Design review of the part built by this model. Coordinates are the model's own, in mm. A direction names the side the tool comes from. Coordinates: 2 decimals unless noted, no trailing zeros. Write each loop counter-clockwise with the first axis right and the second up, starting at its lowest first coordinate (ties: lowest second). Pieces come first, ordered by that corner, then holes. Notation, with made-up numbers: (-24, -26.75) - (15, -26.75) arc R20 ccw to (15, -7.75) - close; hole circle Ø1 at (25, -13.5). An arc over 180 degrees is marked (long way). Answer as CSV lines item,"result". Start each with the question number.
Q1. Clearance check with flat-ended pins moving along their axes: pin 1 (4 mm diameter, centred on x = 18.5, z = -5.5, fed in from -Y); pin 2 (2 mm diameter, centred on x = 8.5, y = 18, fed in from -Z); pin 3 (2 mm diameter, centred on x = -26, y = -31, fed in from +Z); pin 4 (3.5 mm diameter, centred on y = 29, z = -7.5, fed in from -X). State where each tip first meets the part, or that it passes through.
Q2. We need section A-A (x = 17.5). Write out the cut boundary in (y, z), plus the area to 3 significant figures.
Q3. We need section D-D (z = 3.5). Write out the cut boundary in (x, y), plus the area to 3 significant figures.
Q4. For line 1 along X through (y, z) = (17.5, 2.75); line 2 along Y through (x, z) = (15.5, -2.5); line 3 along X through (y, z) = (-26.5, -8), list the stretches that pass through material, from the lowest coordinate up. Write a range as [from, to].
Q5. Machinability: for faces 1 (the face through (25, -10, 3)), 2 (the face through (26, 22.85, -10)), 3 (the face through (9, -32, 0)), 4 (the face through (17, -31, -2)), 5 (the face through (-16.227, 31.299, -9.988)), which of the approach directions +Z, -Z, +X, -X, +Y, -Y give a long, thin tool a straight path to every point of the face, cutting with its end or side? Answer none if there is none.
Q6. We need section C-C (y = -15). Write out the cut boundary in (x, z), plus the area to 3 significant figures.
Q7. We need section B-B (z = -5.72). Write out the cut boundary in (x, y), plus the area to 3 significant figures.
Q8. Mouldability with a two-part tool opening along X and no side actions: class faces 6 (the face through (-26.373, 21.059, 3.131)), 7 (the face through (15, -30, 3)), 8 (the face through (-25, -11, 3)) as pulls with the +X half, pulls with the -X half, needs draft (parallel to the pull), parting line crosses it, or undercut.
from build123d import *

# Parameters (mm, degrees)
SKETCH1_R                                       = 2.85
BOSS_EXTRUDE1_DEPTH                             = 6.35
SKETCH2_W                                       = 25.4
SKETCH2_H                                       = 69.5
SKETCH2_W_2                                     = 14.7
SKETCH2_H_2                                     = 52.8
BOSS_EXTRUDE2_DEPTH                             = 15.578435
CSK_FOR_M8_FLAT_HEAD_MACHINE_SCREW1_D           = 9
CSK_FOR_M8_FLAT_HEAD_MACHINE_SCREW1_DEPTH       = 17.5
CSK_FOR_M8_FLAT_HEAD_MACHINE_SCREW1_CSINK_D     = 17.3
CSK_FOR_M8_FLAT_HEAD_MACHINE_SCREW1_CSINK_ANGLE = 90
CSK_FOR_M8_FLAT_HEAD_MACHINE_SCREW1_TIP         = 2.703872786
SKETCH6_W                                       = 15.578435
SKETCH6_H                                       = 11.9
BOSS_EXTRUDE3_DEPTH                             = 25.572145
SKETCH7_W                                       = 15.578435
SKETCH7_H                                       = 11.9
BOSS_EXTRUDE4_DEPTH                             = 10.937286
SKETCH8_R                                       = 2.5273
CUT_EXTRUDE1_DEPTH                              = 7
SKETCH9_W                                       = 10
SKETCH9_H                                       = 11.9
BOSS_EXTRUDE5_DEPTH                             = 4.972688
SKETCH10_R                                      = 2.5273
CUT_EXTRUDE2_DEPTH                              = 7
SKETCH11_W                                      = 5.3384196
SKETCH11_H                                      = 10
BOSS_EXTRUDE6_DEPTH                             = 5.35
SKETCH14_W                                      = 5.35
SKETCH14_H                                      = 10
CUT_EXTRUDE4_DEPTH                              = 5.33842
SKETCH15_W                                      = 5
SKETCH15_H                                      = 5
SKETCH15_W_2                                    = 8
SKETCH15_H_2                                    = 8
BOSS_EXTRUDE7_DEPTH                             = 8
SKETCH16_R                                      = 2.5273
CUT_EXTRUDE5_DEPTH                              = 7


with BuildPart() as part:
    # Sketch1 → Boss-Extrude1 (new body)
    with BuildSketch(Plane.XY):
        with BuildLine():
            Line((-5, 30), (5, 30))
            Line((5, 30), (25, 30))
            Line((25, 30), (25, 20.148215542))
            Line((25, 20.148215542), (27.91315613, 21.830127018))
            ThreePointArc((27.91315613, 21.830127018), (34.743283149, 19.999999999), (32.91315613, 13.16987298))
            Line((32.91315613, 13.16987298), (25, 8.601210158))
            Line((25, 8.601210158), (25, -30))
            Line((25, -30), (5.102267, -30))
            Line((5.102267, -30), (5.102267, -40))
            ThreePointArc((5.102267, -40), (0.102267, -45), (-4.897733, -40))
            Line((-4.897733, -40), (-4.897733, -30))
            Line((-4.897733, -30), (-25, -30))
            Line((-25, -30), (-25, 8.719297918))
            Line((-25, 8.719297918), (-32.70862213, 13.16987298))
            ThreePointArc((-32.70862213, 13.16987298), (-34.538749149, 19.999999999), (-27.70862213, 21.830127018))
            Line((-27.70862213, 21.830127018), (-25, 20.266303302))
            Line((-25, 20.266303302), (-25, 30))
            Line((-25, 30), (-5, 30))
        make_face()
        with Locations((0.102267, -40)):
            Circle(SKETCH1_R, mode=Mode.SUBTRACT)
        with Locations((30.41315613, 17.499999999)):
            Circle(SKETCH1_R, mode=Mode.SUBTRACT)
        with Locations((-30.20862213, 17.499999999)):
            Circle(SKETCH1_R, mode=Mode.SUBTRACT)
    extrude(amount=BOSS_EXTRUDE1_DEPTH)

    # Sketch2 → Boss-Extrude2 (add)
    with BuildSketch(Plane(origin=(0, 0, 0), x_dir=(-1, 0, 0), z_dir=(0, 0, -1))):
        Rectangle(SKETCH2_W, SKETCH2_H)
        with Locations((0, -3)):
            Rectangle(SKETCH2_W_2, SKETCH2_H_2, mode=Mode.SUBTRACT)
    extrude(amount=BOSS_EXTRUDE2_DEPTH)

    # CSK for M8 Flat Head Machine Screw1
    with Locations(Plane.XY.offset(6.35)):
        with Locations((0, -3)):
            CounterSinkHole(CSK_FOR_M8_FLAT_HEAD_MACHINE_SCREW1_D / 2, CSK_FOR_M8_FLAT_HEAD_MACHINE_SCREW1_CSINK_D / 2, depth=CSK_FOR_M8_FLAT_HEAD_MACHINE_SCREW1_DEPTH, counter_sink_angle=CSK_FOR_M8_FLAT_HEAD_MACHINE_SCREW1_CSINK_ANGLE)
            with Locations((0, 0, -(CSK_FOR_M8_FLAT_HEAD_MACHINE_SCREW1_DEPTH + CSK_FOR_M8_FLAT_HEAD_MACHINE_SCREW1_TIP / 2))):  # 118° drill point
                Cone(0, CSK_FOR_M8_FLAT_HEAD_MACHINE_SCREW1_D / 2, CSK_FOR_M8_FLAT_HEAD_MACHINE_SCREW1_TIP, mode=Mode.SUBTRACT)

    # Sketch6 → Boss-Extrude3 (add)
    with BuildSketch(Plane(origin=(12.7, 0, 0), x_dir=(0, 0, -1), z_dir=(1, 0, 0))):
        with Locations((7.7892175, 28.8)):
            Rectangle(SKETCH6_W, SKETCH6_H)
    extrude(amount=BOSS_EXTRUDE3_DEPTH)

    # Sketch7 → Boss-Extrude4 (add)
    with BuildSketch(Plane.ZY.offset(12.7)):
        with Locations((-7.7892175, 28.8)):
            Rectangle(SKETCH7_W, SKETCH7_H)
    extrude(amount=BOSS_EXTRUDE4_DEPTH)

    # Sketch8 → Cut-Extrude1 (cut)
    with BuildSketch(Plane(origin=(0, 34.75, 0), x_dir=(1, 0, 0), z_dir=(0, 1, 0))):
        with Locations((-18.637286, 9.228435)):
            Circle(SKETCH8_R)
    extrude(amount=-CUT_EXTRUDE1_DEPTH, mode=Mode.SUBTRACT)

    # Sketch9 → Boss-Extrude5 (add)
    with BuildSketch(Plane(origin=(0, 0, -15.578435), x_dir=(-1, 0, 0), z_dir=(0, 0, -1))):
        with Locations((-33.272145, 28.8)):
            Rectangle(SKETCH9_W, SKETCH9_H)
    extrude(amount=BOSS_EXTRUDE5_DEPTH)

    # Sketch10 → Cut-Extrude2 (cut)
    with BuildSketch(Plane(origin=(0, 34.75, 0), x_dir=(1, 0, 0), z_dir=(0, 1, 0))):
        with Locations((33.272145, 14.201123)):
            Circle(SKETCH10_R)
    extrude(amount=-CUT_EXTRUDE2_DEPTH, mode=Mode.SUBTRACT)

    # Sketch11 → Boss-Extrude6 (add)
    with BuildSketch(Plane(origin=(12.7, 0, 0), x_dir=(0, 0, -1), z_dir=(1, 0, 0))):
        with Locations((18.2476448, -8.175)):
            Rectangle(SKETCH11_W, SKETCH11_H)
    extrude(amount=-BOSS_EXTRUDE6_DEPTH)

    # Sketch14 → Cut-Extrude4 (cut)
    with BuildSketch(Plane(origin=(0, 0, -20.9168546), x_dir=(-1, 0, 0), z_dir=(0, 0, -1))):
        with Locations((-10.025, -8.175)):
            Rectangle(SKETCH14_W, SKETCH14_H)
    extrude(amount=-CUT_EXTRUDE4_DEPTH, mode=Mode.SUBTRACT)

    # Sketch15 → Boss-Extrude7 (add)
    with BuildSketch(Plane(origin=(12.7, 0, 0), x_dir=(0, 0, -1), z_dir=(1, 0, 0))):
        with Locations((4.5, 14.55)):
            Rectangle(SKETCH15_W, SKETCH15_H)
        with Locations((4.5, -31.25)):
            Rectangle(SKETCH15_W, SKETCH15_H)
        with Locations((5.72, -8.35)):
            Rectangle(SKETCH15_W_2, SKETCH15_H_2)
    extrude(amount=BOSS_EXTRUDE7_DEPTH)

    # Sketch16 → Cut-Extrude5 (cut)
    with BuildSketch(Plane(origin=(20.7, 0, 0), x_dir=(0, 0, -1), z_dir=(1, 0, 0))):
        with Locations((5.72, -8.35)):
            Circle(SKETCH16_R)
    extrude(amount=-CUT_EXTRUDE5_DEPTH, mode=Mode.SUBTRACT)


solid = part.part
Results list:
1,pin 1,"stops at y = -33.75"
1,pin 2,"stops at z = -15.58"
1,pin 3,"passes through"
1,pin 4,"stops at x = -23.64"
2,outline,"(-33.75, -7) - (-28.75, -7) - (-28.75, -2) - (-33.75, -2) - close; (-30, 0) - (22.85, 0) - (22.85, -15.58) - (34.75, -15.58) - (34.75, 0) - (30, 0) - (30, 6.35) - (-30, 6.35) - close; (-12.35, -9.72) - (-4.35, -9.72) - (-4.35, -1.72) - (-12.35, -1.72) - close; (12.05, -7) - (17.05, -7) - (17.05, -2) - (12.05, -2) - close; hole circle Ø5.05 at (-8.35, -5.72)"
2,area,"660 mm2"
3,outline,"(-32.71, 13.17) - (-25, 8.72) - (-25, -30) - (-4.9, -30) - (-4.9, -40) arc R5 ccw to (5.1, -40) - (5.1, -30) - (25, -30) - (25, 8.6) - (32.91, 13.17) arc R5 ccw to (27.91, 21.83) - (25, 20.15) - (25, 30) - (-25, 30) - (-25, 20.27) - (-27.71, 21.83) arc R5 ccw to start; hole circle Ø5.7 at (-30.21, 17.5); hole circle Ø11.6 at (0, -3); hole circle Ø5.7 at (0.1, -40); hole circle Ø5.7 at (30.41, 17.5)"
3,area,"3,160 mm2"
4,line 1,"x = [-35.21, -33.06], [-27.36, 27.56], [33.26, 35.41]"
4,line 2,"y = [-33.75, -28.75], [-12.35, -4.35], [12.05, 17.05], [22.85, 34.75]"
4,line 3,"x = [-12.7, -7.35], [7.35, 12.7]"
5,face 1,"+Z, -Z, +X, -Y"
5,face 2,"-Z, +X"
5,face 3,"+Z, +X, -Y"
5,face 4,"+X, -Y"
5,face 5,"+Y"
6,outline,"(-25, 0) - (-12.7, 0) - (-12.7, -15.58) - (-7.35, -15.58) - (-7.35, 0) - (7.35, 0) - (7.35, -15.58) - (12.7, -15.58) - (12.7, 0) - (25, 0) - (25, 6.35) - (-25, 6.35) - close"
6,area,"484 mm2"
7,outline,"(-23.64, 22.85) - (-12.7, 22.85) - (-12.7, -34.75) - (12.7, -34.75) - (12.7, -33.75) - (20.7, -33.75) - (20.7, -28.75) - (12.7, -28.75) - (12.7, -12.35) - (20.7, -12.35) - (20.7, -10.88) - (13.7, -10.88) - (13.7, -5.82) - (20.7, -5.82) - (20.7, -4.35) - (12.7, -4.35) - (12.7, 12.05) - (20.7, 12.05) - (20.7, 17.05) - (12.7, 17.05) - (12.7, 22.85) - (38.27, 22.85) - (38.27, 34.75) - (-23.64, 34.75) - close; hole (-7.35, -29.4) - (7.35, -29.4) - (7.35, 23.4) - (-7.35, 23.4) - close"
7,area,"1,530 mm2"
8,face 6,"undercut"
8,face 7,"needs draft"
8,face 8,"pulls with the -X half"
